from build123d import *

# Parameters (mm, degrees)
SKETCH1_W           = 10.16
SKETCH1_H           = 4.953
SKETCH1_W_2         = 7.62
BOSS_EXTRUDE1_DEPTH = 2.4765
CHAMFER2_SIZE       = 3.81


with BuildPart() as part:
    # Sketch1 → Boss-Extrude1 (new body, symmetric)
    with BuildSketch(Plane(origin=(0, 0, 0), x_dir=(0, 0, -1), z_dir=(1, 0, 0))):
        Polygon((45.72, -63.246), (45.72, -16.5735), (38.1, -16.5735), (38.1, -11.6205), (45.72, -11.6205), (45.72, 11.6205), (38.1, 11.6205), (38.1, 16.5735), (45.72, 16.5735), (45.72, 63.246), (-16.571856626, 63.246), (-16.571856626, 16.5735), (-39.096447575, 16.5735), (-43.495856626, 14.0335), (-43.495856626, -14.0335), (-39.096447575, -16.5735), (-16.571856626, -16.5735), (-16.571856626, -63.246), align=None)
        with Locations((33.02, -52.0065)):
            Rectangle(SKETCH1_W, SKETCH1_H, mode=Mode.SUBTRACT)
        with Locations((33.02, 52.0065)):
            Rectangle(SKETCH1_W, SKETCH1_H, mode=Mode.SUBTRACT)
        with Locations((-3.871856626, 52.0065)):
            Rectangle(SKETCH1_W, SKETCH1_H, mode=Mode.SUBTRACT)
        with Locations((-3.871856626, -52.0065)):
            Rectangle(SKETCH1_W, SKETCH1_H, mode=Mode.SUBTRACT)
        with Locations((7.62, 14.097)):
            Rectangle(SKETCH1_W_2, SKETCH1_H, mode=Mode.SUBTRACT)
        with Locations((7.62, -14.097)):
            Rectangle(SKETCH1_W_2, SKETCH1_H, mode=Mode.SUBTRACT)
    extrude(amount=BOSS_EXTRUDE1_DEPTH, both=True)

    # Chamfer2
    chamfer2_edges = [part.edges().sort_by_distance(p)[0] for p in [
        (0, -63.246, -45.72),
        (0, -63.246, 16.571856626),
        (0, 63.246, 16.571856626),
        (0, 63.246, -45.72),
    ]]
    chamfer(chamfer2_edges, length=CHAMFER2_SIZE)


solid = part.part
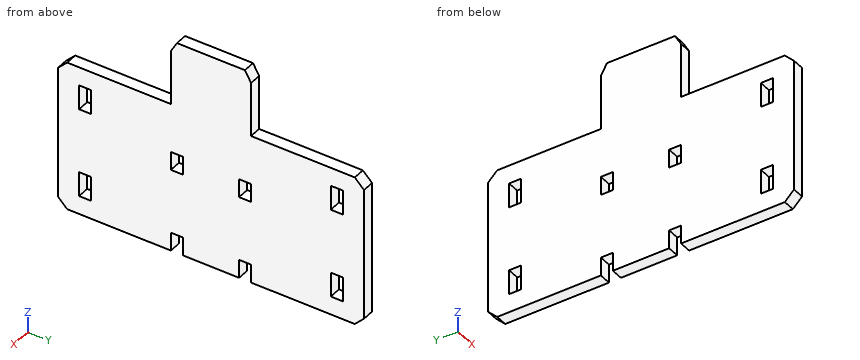
Input: part model. Units: mm. Frame: model coordinates. Round coordinates to 2 decimals unless told otherwise and drop trailing zeros. Write each loop counter-clockwise with the first axis right and the second up, starting at its lowest first coordinate (ties: lowest second). Pieces come first, ordered by that corner, then holes.
1) Contact query for flat-ended pins moving along their axis: P1, Ø2.5, axis at x = 0.5, z = 32.5, coming from the -Y side; P2, Ø1.5, axis at x = 0, y = 51, coming from the +Z side; P3, Ø1.5, axis at x = 0.5, y = 14.5, coming from the -Z side. Output: stop coordinate, or through.
2) Cut plane C-C (z = 19). Return the cut outline in (x, y), then the cut area to 3 significant figures.
3) Ray query, L1, parallel to Z at x = 2.05, y = 53; L2, parallel to Y at x = -1.8, z = 5.5; L3, parallel to Y at x = 1.25, z = -4. Return the intervals inside material, ascending.
4) Cut plane B-B (x = 0.85). Count the separate pieces of the cut face and the enclosed holes in it, then the cut area to 3 significant figures.
5) Cut plane A-A (y = -52.5). Return the cut outline in (x, z), then the cut area to 3 significant figures.
Geometry says:
1. P1: stops at y = -16.57
1. P2: stops at z = 16.57
1. P3: stops at z = -38.1
2. outline: (-2.48, -16.57) - (2.48, -16.57) - (2.48, 16.57) - (-2.48, 16.57) - close
2. area: 164 mm2
3. L1: z = -45.72 to -38.1, -27.94 to -1.21, 8.95 to 16.57
3. L2: y = -63.25 to -54.48, -49.53 to 49.53, 54.48 to 63.25
3. L3: y = -63.25 to -16.57, -11.62 to 11.62, 16.57 to 63.25
4. separate pieces: 1
4. enclosed holes: 6
4. area: 8,380 mm2
5. outline: (-2.48, -45.72) - (2.48, -45.72) - (2.48, -38.1) - (-2.48, -38.1) - close; (-2.48, -27.94) - (2.48, -27.94) - (2.48, -1.21) - (-2.48, -1.21) - close; (-2.48, 8.95) - (2.48, 8.95) - (2.48, 16.57) - (-2.48, 16.57) - close
5. area: 208 mm2
